The listing builds one solid part. Answer for the finished solid, in the listing's coordinates (mm). Give positions to 0.01 mm unless a question says otherwise; leave off trailing zeros. Write each loop counter-clockwise with the first axis right and the second up, starting at its lowest first coordinate (ties: lowest second). Pieces come first, ordered by that corner, then holes.
Autodesk Inventor part; units mm, degrees
ref_plane "YZ Plane" through (0, 0, 0) normal (1, 0, 0) x (0, 1, 0)
ref_plane "XZ Plane" through (0, 0, 0) normal (0, 1, 0) x (-1, 0, 0)
ref_plane "XY Plane" through (0, 0, 0) normal (0, 0, 1) x (1, 0, 0)
sketch "Sketch1" plane through (0, 0, 0) normal (0, 0, 1) x (1, 0, 0)
  line L0 (0, 0) -> (0, 38.1)
  line L1 (0, 38.1) -> (114.3, 38.1)
  line L2 (114.3, 38.1) -> (114.3, 0)
  line L3 (0, 0) -> (114.3, 0)
  dimension "d0" = 38.1
  dimension "d1" = 114.3
extrude "Extrusion1" add sketch "Sketch1" along normal blind 3.175
sketch "Sketch2" plane through (0, 0, 3.175) normal (0, 0, 1) x (1, 0, 0)
  line L0 (114.3, 0) -> (114.3, 38.1)
  line L1 (114.3, 38.1) -> (0, 38.1)
  circle A0 centre (57.15, 19.05) radius 2.54
  line L2 (0, 38.1) -> (0, 0)
  circle A1 centre (19.05, 19.05) radius 3.175
  circle A2 centre (95.25, 19.05) radius 3.175
  dimension "d4" = 5.08
  dimension "d5" = 19.05
  dimension "d6" = 57.15
  dimension "d9" = 6.35
  dimension "d10" = 6.35
  dimension "d11" = 19.05
  dimension "d12" = 19.05
extrude "Extrusion3" cut sketch "Sketch2" against normal blind 25.4
properties part number "PistonPlate_v1"
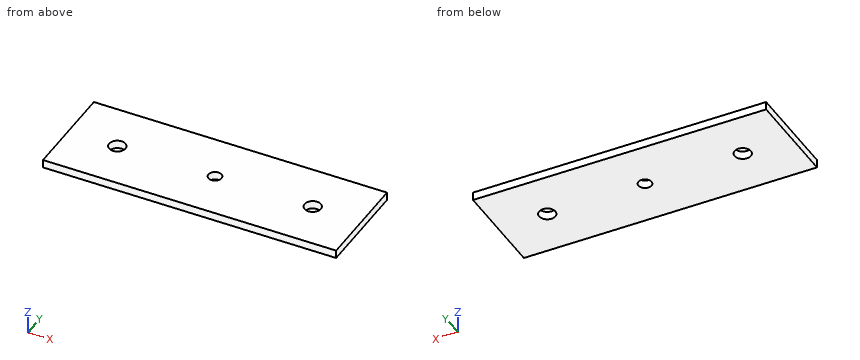
Item 1: A cutting plane is placed at A-A, the plane x = 57.15. Give the vertices of the cut face in (y, z) (3 decimals), plus the area to 3 significant figures.
Conclusion:
outline: (0, 0) - (16.51, 0) - (16.51, 3.175) - (0, 3.175) - close; (21.59, 0) - (38.1, 0) - (38.1, 3.175) - (21.59, 3.175) - close
area: 105 mm2
Item 2: A cutting plane is placed at D-D, the plane x = 95.25. Give the vertices of the cut face in (y, z) (3 decimals).
Conclusion:
outline: (0, 0) - (15.875, 0) - (15.875, 3.175) - (0, 3.175) - close; (22.225, 0) - (38.1, 0) - (38.1, 3.175) - (22.225, 3.175) - close
Item 3: Consider probe 1 along Y at (x, z) = (57.15, 2.3); probe 2 along Y at (x, z) = (95.25, 1.45) (3 decimals); probe 3 along X at (y, z) = (19.5, 1.3). Determine where each line is inside the solid, lowest interval first.
Conclusion:
probe 1: y = 0 to 16.51, 21.59 to 38.1
probe 2: y = 0 to 15.875, 22.225 to 38.1
probe 3: x = 0 to 15.91, 22.19 to 54.65, 59.65 to 92.11, 98.39 to 114.3
Item 4: A cutting plane is placed at B-B, the plane y = 19.05. Give the vertices of the cut face in (x, z) (3 decimals).
Conclusion:
outline: (0, 0) - (15.875, 0) - (15.875, 3.175) - (0, 3.175) - close; (22.225, 0) - (54.61, 0) - (54.61, 3.175) - (22.225, 3.175) - close; (59.69, 0) - (92.075, 0) - (92.075, 3.175) - (59.69, 3.175) - close; (98.425, 0) - (114.3, 0) - (114.3, 3.175) - (98.425, 3.175) - close
Item 5: A cutting plane is placed at C-C, the plane z = 2.55. Give the vertices of the cut face in (x, y) (3 decimals), plus the area to 3 significant figures.
Conclusion:
outline: (0, 0) - (114.3, 0) - (114.3, 38.1) - (0, 38.1) - close; hole circle Ø6.35 at (19.05, 19.05); hole circle Ø5.08 at (57.15, 19.05); hole circle Ø6.35 at (95.25, 19.05)
area: 4,270 mm2
